```python
from build123d import *

# Parameters (mm, degrees)
BOSS_EXTRUDE1_DEPTH     = 10
CUT_EXTRUDE1_DEPTH      = 158.241851935
CUT_EXTRUDE1_DEPTH_BACK = 158.241851935
SKETCH4_R               = 2


with BuildPart() as part:
    # Sketch1 → Boss-Extrude1 (new body)
    with BuildSketch(Plane.XY):
        Polygon((0, 0), (0, 60), (145, 60), (145, 0), (135, 0), (135, 50), (10, 50), (10, 0), align=None)
    extrude(amount=BOSS_EXTRUDE1_DEPTH)

    # Sketch4 → Cut-Extrude1 (cut, two sides: drawn at the far end of the back side and taken through both)
    with BuildSketch(Plane(origin=(145, 0, 0), x_dir=(0, 0, -1), z_dir=(1, 0, 0)).offset(-CUT_EXTRUDE1_DEPTH_BACK)):
        with Locations((-5, 10)):
            Circle(SKETCH4_R)
        with Locations((-5, 40)):
            Circle(SKETCH4_R)
    extrude(amount=CUT_EXTRUDE1_DEPTH + CUT_EXTRUDE1_DEPTH_BACK, mode=Mode.SUBTRACT)


solid = part.part
```
Part model, mm, in its own coordinate system. A direction names the side the tool comes from. Give positions to 0.01 mm unless a question says otherwise; leave off trailing zeros. Write each loop counter-clockwise with the first axis right and the second up, starting at its lowest first coordinate (ties: lowest second). Pieces come first, ordered by that corner, then holes. Notation, with made-up numbers: M -36.5,18 L 17.5,18 A12 ccw 17.5,32 Z; hole C 35.5,77 d7. An arc over 180 degrees is marked long. Use CSV: the item, a comma, the result in double quotes.
Item 1: Slice it at A-A on y = 20.5. Write the cut outline in (x, z), plus the area to 3 significant figures.
Taken from the geometry:
outline,"M 0,0 L 10,0 L 10,10 L 0,10 Z; M 135,0 L 145,0 L 145,10 L 135,10 Z"
area,"200 mm²"
Item 2: Drill centre lines: probe 1 along Y at (x, z) = (6.5, 5); probe 2 along X at (y, z) = (17, 9); probe 3 along Z at (x, y) = (140.75, 40). Where is each one in solid material? Low to high.
Taken from the geometry:
probe 1,"y = 0 to 8, 12 to 38, 42 to 60"
probe 2,"x = 0 to 10, 135 to 145"
probe 3,"z = 0 to 3, 7 to 10"
Item 3: Slice it at C-C on z = 5. Write the cut outline in (x, y), plus the area to 3 significant figures.
Taken from the geometry:
outline,"M 0,0 L 10,0 L 10,8 L 0,8 Z; M 0,12 L 10,12 L 10,38 L 0,38 Z; M 0,42 L 10,42 L 10,50 L 135,50 L 135,42 L 145,42 L 145,60 L 0,60 Z; M 135,0 L 145,0 L 145,8 L 135,8 Z; M 135,12 L 145,12 L 145,38 L 135,38 Z"
area,"2,290 mm²"
Item 4: Slice it at D-D on x = 96. Write the cut outline in (y, z).
Taken from the geometry:
outline,"M 50,0 L 60,0 L 60,10 L 50,10 Z"
Item 5: Pull direction Z, two halves, no side cores. Call faces 3 (the face through (140, 38, 5)), 4 (the face through (5, 0, 5)), 5 (the face through (73.5, 50.4, 10)): +Z half, -Z half, draft (parallel to the pull), parting line (faces both ways), or undercut.
Taken from the geometry:
face 3,"undercut"
face 4,"draft"
face 5,"+Z half"
Item 6: Slice it at B-B on y = 10. Write the cut outline in (x, z).
Taken from the geometry:
outline,"M 0,0 L 10,0 L 10,3 L 0,3 Z; M 0,7 L 10,7 L 10,10 L 0,10 Z; M 135,0 L 145,0 L 145,3 L 135,3 Z; M 135,7 L 145,7 L 145,10 L 135,10 Z"
Item 7: Pin check, flat tips, straight feed: P1, Ø4.5, axis at y = 40, z = 5, coming from the -X side; P2, Ø3.5, axis at y = 10, z = 5, coming from the -X side; P3, Ø5, axis at x = 89.5, z = 6, coming from the -Y side. Stop position of each tip, or through.
Taken from the geometry:
P1,"stops at x = 0"
P2,"passes through"
P3,"stops at y = 50"
Item 8: Which spindle directions (+Z, -Z, +X, -X, +Y, -Y) get a long thin tool onto all of the face, cutting with end or side? Do faces 1 (the face through (145, 30, 5)), 2 (the face through (135, 25, 5)). Say none if no direction does.
Taken from the geometry:
face 1,"+Z, -Z, +X, +Y, -Y"
face 2,"+Z, -Z, -Y"
